The model under review builds one solid part; all positions refer to its coordinate system, in mm. A direction names the side the tool comes from. Round coordinates to 2 decimals unless told otherwise and drop trailing zeros. Loops run counter-clockwise (first coordinate to the right, second up) from the corner with the lowest first, then second, coordinate; pieces in that order, holes last. Notation, with made-up numbers: M 47.5,23 L 87.5,23 A24 cw 87.5,61 Z; hole C 14.5,35.25 d11. An arc over 180 degrees is marked long. One line per question, with ' | ' between items.
from build123d import *

# Parameters (mm, degrees)
SKETCH_1_W                = 30
SKETCH_1_H                = 10
EXTRUDE_1_DEPTH           = 5
SKETCH_4_W                = 6
SKETCH_4_H                = 3
CUT_EXTRUDE_1_DEPTH       = 17.583123952
HOLE_WIZARD_1_D           = 3.4
HOLE_WIZARD_1_CBORE_D     = 6
HOLE_WIZARD_1_CBORE_DEPTH = 3.4


with BuildPart() as part:
    # 草图1 → 凸台-拉伸1 (new body)
    with BuildSketch(Plane(origin=(0, 0, 0), x_dir=(0, 0, -1), z_dir=(1, 0, 0))):
        Rectangle(SKETCH_1_W, SKETCH_1_H)
    extrude(amount=EXTRUDE_1_DEPTH)

    # 草图4 → 切除-拉伸1 (cut, through all)
    with BuildSketch(Plane(origin=(5, 0, 0), x_dir=(0, 0, -1), z_dir=(1, 0, 0))):
        with Locations((12, 3.5)):
            Rectangle(SKETCH_4_W, SKETCH_4_H)
        with Locations((-12, 3.5)):
            Rectangle(SKETCH_4_W, SKETCH_4_H)
    extrude(amount=-CUT_EXTRUDE_1_DEPTH, mode=Mode.SUBTRACT)

    # 打孔尺寸根据内六角圆柱头螺钉的类型1 (through all)
    with Locations(Plane(origin=(5, 0, 0), x_dir=(0, 0, -1), z_dir=(1, 0, 0))):
        with Locations((-7.5, -1.5), (7.5, -1.5)):
            CounterBoreHole(HOLE_WIZARD_1_D / 2, HOLE_WIZARD_1_CBORE_D / 2, HOLE_WIZARD_1_CBORE_DEPTH)


solid = part.part
1) Mouldability with a two-part tool opening along Z and no side actions: class faces 1 (the flat face through (3, 2, -12)), 2 (the flat face through (3, 3, 9)), 3 (the flat face through (2, -2, -15)), 4 (the cylindrical face through (3.32, -2.65, -10.27)) as +Z half, -Z half, draft (parallel to the pull), parting line (faces both ways), or undercut.
Output values:
face 1: draft | face 2: +Z half | face 3: -Z half | face 4: undercut
2) Insertion check: P1, Ø0.9, axis at x = 1.5, y = 3, coming from the -Z side; P2, Ø1.8, axis at y = -1.5, z = 8.5, coming from the +X side. Each pin has a flat end and moves straight along its axis. Give the tip position at first contact, or say it passes through.
Output values:
P1: stops at z = -9 | P2: stops at x = 1.6
3) For line 1 (Z direction, x = 0.45, y = -0.5); line 2 (Z direction, x = 2.15, y = 0.5); line 3 (Z direction, x = 2.4, y = 3.5), list the stretches that pass through material, from the lowest coordinate up.
Output values:
line 1: z = -15 to -8.87, -6.13 to 6.13, 8.87 to 15 | line 2: z = -15 to -9.74, -5.26 to 5.26, 9.74 to 15 | line 3: z = -9 to 9
4) Add section D-D on y = 2.5. State the section outline as (x, z) points.
Output values:
outline: M 0,-9 L 5,-9 L 5,9 L 0,9 Z
5) Add section A-A on z = -7.5. State the section outline as (x, y) points, then the cut area to 3 significant figures.
Output values:
outline: M 0,-5 L 5,-5 L 5,-4.5 L 1.6,-4.5 L 1.6,-3.2 L 0,-3.2 Z; M 0,0.2 L 1.6,0.2 L 1.6,1.5 L 5,1.5 L 5,5 L 0,5 Z | area: 24.2 mm²
6) Machinability: for faces 5 (the flat face through (1.6, -3, -9)), 6 (the cylindrical face through (0.79, -1.43, -9.2)), 7 (the flat face through (3, 3, -9)), 8 (the flat face through (3, 2, 12)), which of the approach directions +Z, -Z, +X, -X, +Y, -Y give a long, thin tool a straight path to every point of the face, cutting with its end or side? Answer none if there is none.
Output values:
face 5: +X | face 6: +X, -X | face 7: -Z, +X, -X, +Y | face 8: +Z, +X, -X, +Y
7) Add section B-B on x = 2.2. State the section outline as (y, z) points, then the cut area to 3 significant figures.
Output values:
outline: M -5,-15 L 2,-15 L 2,-9 L 5,-9 L 5,9 L 2,9 L 2,15 L -5,15 Z; hole C -1.5,-7.5 d6; hole C -1.5,7.5 d6 | area: 207 mm²
8) Add section C-C on y = -2.25. State the section outline as (x, z) points.
Output values:
outline: M 0,-15 L 5,-15 L 5,-10.4 L 1.6,-10.4 L 1.6,-9.03 L 0,-9.03 Z; M 0,-5.97 L 1.6,-5.97 L 1.6,-4.6 L 5,-4.6 L 5,4.6 L 1.6,4.6 L 1.6,5.97 L 0,5.97 Z; M 0,9.03 L 1.6,9.03 L 1.6,10.4 L 5,10.4 L 5,15 L 0,15 Z
